Input: part model. Units: mm. Frame: model coordinates. Give positions to 0.01 mm unless a question says otherwise; leave off trailing zeros. Loops run counter-clockwise (first coordinate to the right, second up) from the corner with the lowest first, then second, coordinate; pieces in that order, holes last. Notation, with made-up numbers: (14, 48.5) - (59, 48.5) arc R29 cw to (59, 87.5) - close; hole circle Ø9 at (-4.75, 73). An arc over 180 degrees is marked (long way). Answer as a JSON object with one key per item and string values. Group by question number.
(1) Pin query (flat end, axial travel): P1, Ø4, axis at y = 47.5, z = 4, coming from the -X side; P2, Ø5, axis at x = 4.5, y = 46, coming from the -Z side; P3, Ø10, axis at y = 33.5, z = -8, coming from the +X side. Return the tip coordinate at first contact, or that it passes through.
(2) Section query B-B (x = 0). Return loops of the section in (y, z).
(3) Section query C-C (y = 28). Return loops of the section in (x, z), plus the area to 3 significant figures.
(4) Material intervals for L1, parallel to X at y = 51, z = 0; L2, parallel to Z at x = -4, y = 38; L3, parallel to X at y = 14.5, z = -3, sorted ascending.
(5) Mould query, pull axis X, two halves, no side actions, for faces 1 (the cylindrical face through (-2.43, 37.34, 5.86)), 2 (the cylindrical face through (-10.648, 37.336, -13.887)), 3 (the flat face through (0, 75.722, 7)). Classes: +X half, -X half, draft (parallel to the pull), parting line (faces both ways), or undercut.
(6) Section query A-A (z = 0). Return loops of the section in (x, y).
```python
from build123d import *

# Parameters (mm, degrees)
SKETCH1_R           = 17.5
BOSS_EXTRUDE1_DEPTH = 75.721727
SKETCH2_R           = 6.345843567
CUT_EXTRUDE1_DEPTH  = 80.6635421
CHAMFER1_SIZE       = 0.350058


with BuildPart() as part:
    # Sketch1 → Boss-Extrude1 (new body)
    with BuildSketch(Plane(origin=(0, 0, 0), x_dir=(1, 0, 0), z_dir=(0, 1, 0))):
        with Locations(Location((0, 0, 0), (0, 0, 270))):
            Circle(SKETCH1_R)
    extrude(amount=BOSS_EXTRUDE1_DEPTH)

    # Sketch2 → Cut-Extrude1 (cut, through all)
    with BuildSketch(Plane(origin=(0, 0, 0), x_dir=(1, 0, 0), z_dir=(0, 1, 0))):
        with Locations(Location((0, 0, 0), (0, 0, 270))):
            Circle(SKETCH2_R)
    extrude(amount=CUT_EXTRUDE1_DEPTH, mode=Mode.SUBTRACT)

    # Chamfer1
    chamfer1_edges = [part.edges().sort_by_distance(p)[0] for p in [
        (0, 0, -17.5),
        (0, 75.721727, -17.5),
        (0, 0, -6.345843567),
        (0, 75.721727, -6.345843567),
    ]]
    chamfer(chamfer1_edges, length=CHAMFER1_SIZE)


solid = part.part
```
Recorded:
{
 "1": {"P1": "stops at x = -17.39", "P2": "stops at z = -17.39", "P3": "stops at x = 17.24"},
 "2": {"outline": "(0, -17.15) - (0.35, -17.5) - (75.37, -17.5) - (75.72, -17.15) - (75.72, -6.7) - (75.37, -6.35) - (0.35, -6.35) - (0, -6.7) - close; (0, 6.7) - (0.35, 6.35) - (75.37, 6.35) - (75.72, 6.7) - (75.72, 17.15) - (75.37, 17.5) - (0.35, 17.5) - (0, 17.15) - close"},
 "3": {"outline": "circle Ø35 at (0, 0); hole circle Ø12.69 at (0, 0)", "area": "836 mm^2"},
 "4": {"L1": "x = -17.5 to -6.35, 6.35 to 17.5", "L2": "z = -17.04 to -4.93, 4.93 to 17.04", "L3": "x = -17.24 to -5.59, 5.59 to 17.24"},
 "5": {"face 1": "undercut", "face 2": "parting line", "face 3": "draft"},
 "6": {"outline": "(-17.5, 0.35) - (-17.15, 0) - (-6.7, 0) - (-6.35, 0.35) - (-6.35, 75.37) - (-6.7, 75.72) - (-17.15, 75.72) - (-17.5, 75.37) - close; (6.35, 0.35) - (6.7, 0) - (17.15, 0) - (17.5, 0.35) - (17.5, 75.37) - (17.15, 75.72) - (6.7, 75.72) - (6.35, 75.37) - close"}
}
